The model under review builds one solid part; all positions refer to its coordinate system, in mm. A direction names the side the tool comes from. Coordinates: 2 decimals unless noted, no trailing zeros. Loops run counter-clockwise (first coordinate to the right, second up) from the corner with the lowest first, then second, coordinate; pieces in that order, holes last. Notation, with made-up numbers: (9, -6) - (61, -6) arc R5 ccw to (61, 3) - close; hole circle Ø3 at (-0.5, 8). An arc over 180 degrees is marked (long way). Answer in a Markdown table with one row per item. Add a question column.
(1) For line 1 along X through (y, z) = (-0.1, 11.25); line 2 along Y through (x, z) = (-0.75, 10.5); line 3 along X through (y, z) = (-0.5, 8), list the stretches that pass through material, from the lowest coordinate up.
(2) Machinability: for faces 1 (the flat face through (1, -1, 13)), 2 (the cylindrical face through (-3, 0.1, 13.6)), which of the approach directions +Z, -Z, +X, -X, +Y, -Y give a long, thin tool a straight path to every point of the face, cutting with its end or side? Answer none if there is none.
(3) We need section A-A on z = 1. Write out the cut boundary in (x, y).
(4) For P1, Ø3, axis at y = 0.5, z = 10, coming from the +X side; P2, Ø2, axis at x = 1, z = 9, coming from the -Y side; P3, Ø3, axis at x = 0.5, z = 10.5, coming from the +Y side, all flat-tipped, find the tip position at first contact; note any pin that passes through.
from build123d import *

# Parameters (mm, degrees)
SKETCH1_R           = 1.25
BOSS_EXTRUDE1_DEPTH = 16
SKETCH2_R           = 3
BOSS_EXTRUDE2_DEPTH = 3
FILLET1_R           = 2
CHAMFER1_SIZE       = 0.256


with BuildPart() as part:
    # Sketch1 → Boss-Extrude1 (new body)
    with BuildSketch(Plane.XY):
        Circle(SKETCH1_R)
    extrude(amount=BOSS_EXTRUDE1_DEPTH)

    # Sketch2 → Boss-Extrude2 (add)
    with BuildSketch(Plane.XY.offset(16)):
        Circle(SKETCH2_R)
    extrude(amount=-BOSS_EXTRUDE2_DEPTH)

    # Fillet1
    fillet1_edges = [part.edges().sort_by_distance(p)[0] for p in [
        (-3, 0, 16),
    ]]
    fillet(fillet1_edges, radius=FILLET1_R)

    # Chamfer1
    chamfer1_edges = [part.edges().sort_by_distance(p)[0] for p in [
        (-3, 0, 13),
    ]]
    chamfer(chamfer1_edges, length=CHAMFER1_SIZE)


solid = part.part
Outcome:
| question | item | result |
|---|---|---|
| 1 | line 1 | -1.25 to 1.25 |
| 1 | line 2 | -1 to 1 |
| 1 | line 3 | -1.15 to 1.15 |
| 2 | face 1 | -Z |
| 2 | face 2 | +Z, -Z |
| 3 | outline | circle Ø2.5 at (0, 0) |
| 4 | P1 | x = 1.25 |
| 4 | P2 | y = -1.25 |
| 4 | P3 | y = 1.25 |
